```python
from build123d import *

# Parameters (mm, degrees)
SKETCH1_W           = 154
SKETCH1_H           = 41
BOSS_EXTRUDE1_DEPTH = 2
SKETCH2_R           = 1.5
CUT_EXTRUDE1_DEPTH  = 204
SKETCH3_R           = 1.5
BOSS_EXTRUDE2_DEPTH = 154
SKETCH4_W           = 12
SKETCH4_H           = 23.161381141
SKETCH4_W_2         = 3
SKETCH4_H_2         = 18.642875374
SKETCH4_H_3         = 14.783247827
SKETCH4_W_3         = 14
SKETCH4_H_4         = 17.598544921
SKETCH4_H_5         = 27.804183012
CUT_EXTRUDE2_DEPTH  = 204
SKETCH5_W           = 3
SKETCH5_H           = 13.316127407
CUT_EXTRUDE3_DEPTH  = 5
SKETCH6_W           = 8
SKETCH6_H           = 34.567606234
CUT_EXTRUDE4_DEPTH  = 1
SKETCH7_W           = 10.416873331
SKETCH7_H           = 25.160109374
BOSS_EXTRUDE3_DEPTH = 1
FILLET1_R           = 10
BOSS_EXTRUDE4_DEPTH = 2
FILLET2_R           = 2
FILLET3_R           = 2
FILLET4_R           = 0.2


with BuildPart() as part:
    # Sketch1 → Boss-Extrude1 (new body)
    with BuildSketch(Plane.XY):
        with Locations((46, -32.5)):
            Rectangle(SKETCH1_W, SKETCH1_H)
    extrude(amount=BOSS_EXTRUDE1_DEPTH)

    # Sketch2 → Cut-Extrude1 (cut)
    with BuildSketch(Plane.ZY.offset(31)):
        with Locations((-1, -17)):
            Circle(SKETCH2_R)
    extrude(amount=-CUT_EXTRUDE1_DEPTH, mode=Mode.SUBTRACT)

    # Sketch3 → Boss-Extrude2 (add)
    with BuildSketch(Plane.ZY.offset(31)):
        with BuildLine():
            Line((-2.639541446, -19.403784927), (0, -21.185182296))
            Line((0, -21.185182296), (0, -19.715731065))
            ThreePointArc((0, -19.715731065), (1.882746452, -17), (0, -14.284268935))
            Line((0, -14.284268935), (0, -13.471330145))
            Line((0, -13.471330145), (-2.092481561, -14.306696319))
            ThreePointArc((-2.092481561, -14.306696319), (-3.900693524, -16.690526404), (-2.639541446, -19.403784927))
        make_face()
        with Locations((-1.017253548, -17)):
            Circle(SKETCH3_R, mode=Mode.SUBTRACT)
    extrude(amount=-BOSS_EXTRUDE2_DEPTH)

    # Sketch4 → Cut-Extrude2 (cut)
    with BuildSketch(Plane(origin=(0, 0, 0), x_dir=(-1, 0, 0), z_dir=(0, 0, -1))):
        with Locations((22, -9.604491726)):
            Rectangle(SKETCH4_W, SKETCH4_H)
        with Locations((-80.5, -11.863744609)):
            Rectangle(SKETCH4_W_2, SKETCH4_H_2)
        with Locations((-114, -13.793558383)):
            Rectangle(SKETCH4_W, SKETCH4_H_3)
        with Locations((-103.5, -11.863744609)):
            Rectangle(SKETCH4_W_2, SKETCH4_H_2)
        with Locations((-92, -12.385909835)):
            Rectangle(SKETCH4_W_3, SKETCH4_H_4)
        with Locations((-69, -12.385909835)):
            Rectangle(SKETCH4_W_3, SKETCH4_H_4)
        with Locations((-57.5, -11.863744609)):
            Rectangle(SKETCH4_W_2, SKETCH4_H_2)
        with Locations((-46, -12.385909835)):
            Rectangle(SKETCH4_W_3, SKETCH4_H_4)
        with Locations((-34.5, -11.863744609)):
            Rectangle(SKETCH4_W_2, SKETCH4_H_2)
        with Locations((-23, -12.385909835)):
            Rectangle(SKETCH4_W_3, SKETCH4_H_4)
        with Locations((-11.5, -11.863744609)):
            Rectangle(SKETCH4_W_2, SKETCH4_H_2)
        with Locations((0, -12.385909835)):
            Rectangle(SKETCH4_W_3, SKETCH4_H_4)
        with Locations((11.5, -7.28309079)):
            Rectangle(SKETCH4_W_2, SKETCH4_H_5)
    extrude(amount=CUT_EXTRUDE2_DEPTH, mode=Mode.SUBTRACT)

    # Sketch5 → Cut-Extrude3 (cut)
    with BuildSketch(Plane(origin=(0, 0, 0), x_dir=(-1, 0, 0), z_dir=(0, 0, -1))):
        with Locations((-80.5, -11.44429523)):
            Rectangle(SKETCH5_W, SKETCH5_H)
        with Locations((-103.5, -11.44429523)):
            Rectangle(SKETCH5_W, SKETCH5_H)
        with Locations((-57.5, -11.44429523)):
            Rectangle(SKETCH5_W, SKETCH5_H)
        with Locations((-34.5, -11.44429523)):
            Rectangle(SKETCH5_W, SKETCH5_H)
        with Locations((-11.5, -11.44429523)):
            Rectangle(SKETCH5_W, SKETCH5_H)
        with Locations((11.5, -11.44429523)):
            Rectangle(SKETCH5_W, SKETCH5_H)
    extrude(amount=-CUT_EXTRUDE3_DEPTH, mode=Mode.SUBTRACT)

    # Sketch6 → Cut-Extrude4 (cut)
    with BuildSketch(Plane(origin=(0, 0, 0), x_dir=(-1, 0, 0), z_dir=(0, 0, -1))):
        with Locations((-46, -29.283803117)):
            Rectangle(SKETCH6_W, SKETCH6_H)
    extrude(amount=-CUT_EXTRUDE4_DEPTH, mode=Mode.SUBTRACT)

    # Sketch7 → Boss-Extrude3 (add)
    with BuildSketch(Plane(origin=(0, 0, 0), x_dir=(-1, 0, 0), z_dir=(0, 0, -1))):
        with Locations((-46.159585617, -34.952904223)):
            Rectangle(SKETCH7_W, SKETCH7_H)
    extrude(amount=BOSS_EXTRUDE3_DEPTH)

    # Fillet1
    # the kernel refuses this fillet: 10 mm, written as the material it takes off along each edge
    with BuildSketch(Plane(origin=(40.951148952, -11.475602177, -1), x_dir=(0, 0, 1), z_dir=(0, -1, 0)), Plane(origin=(51.368022283, -58.430206269, -1), x_dir=(0, 0, 1), z_dir=(0, 1, 0))) as fillet1_piece_1:
        with BuildLine():
            CenterArc((10, -4.358898944), FILLET1_R, 154.158067237, 25.841932763)
            Line((0, -4.358898944), (-0.2, -4.358898944))
            Line((-0.2, -4.358898944), (-0.2, 0))
            Line((-0.2, 0), (0, 0.2))
            ThreePointArc((0, 0.2), (0.5, 0.2), (0.82, 0.087177979))
            Line((0.82, 0.087177979), (1, 0))
        make_face()
    extrude(amount=46.954604092, mode=Mode.SUBTRACT)
    with BuildSketch(Plane(origin=(30.053901593, -47.53295891, -1), x_dir=(0, 0, 1), z_dir=(1, 0, 0))) as fillet1_piece_2:
        with BuildLine():
            CenterArc((10, -4.358898944), FILLET1_R, 154.158067237, 25.841932763)
            Line((0, -4.358898944), (-0.2, -4.358898944))
            Line((-0.2, -4.358898944), (-0.2, 0))
            Line((-0.2, 0), (0, 0.2))
            ThreePointArc((0, 0.2), (0.5, 0.2), (0.82, 0.087177979))
            Line((0.82, 0.087177979), (1, 0))
        make_face()
    extrude(amount=32.211368048, mode=Mode.SUBTRACT)

    # Sketch8 → Boss-Extrude4 (add)
    with BuildSketch(Plane.XY.offset(2)):
        with BuildLine():
            Line((42.287250182, -53), (49.726428085, -53))
            Line((49.726428085, -53), (49.726428085, -55.335034312))
            ThreePointArc((49.726428085, -55.335034312), (46.006839134, -57.703773476), (42.287250182, -55.335034312))
            Line((42.287250182, -55.335034312), (42.287250182, -53))
        make_face()
    extrude(amount=-BOSS_EXTRUDE4_DEPTH)

    # Fillet2
    fillet2_edges = [part.edges().sort_by_distance(p)[0] for p in [
        (49.726428085, -53, 1),
        (42.287250182, -53, 1),
    ]]
    fillet(fillet2_edges, radius=FILLET2_R)

    # Fillet3
    fillet3_edges = [part.edges().sort_by_distance(p)[0] for p in [
        (42.287250182, -55.335034312, 1),
        (49.726428085, -55.335034312, 1),
    ]]
    fillet(fillet3_edges, radius=FILLET3_R)

    # Fillet4
    fillet4_edges = [part.edges().sort_by_distance(p)[0] for p in [
        (123, -32.5, 2),
        (87.363214043, -53, 2),
        (-31, -32.5, 2),
        (-22, -12, 2),
        (0, -12, 2),
        (23, -12, 2),
        (46, -12, 2),
        (69, -12, 2),
        (92, -12, 2),
        (114, -12, 2),
        (-13, -15.051179467, 2),
        (-11.5, -18.102358934, 2),
        (-10, -15.051179467, 2),
        (10, -15.051179467, 2),
        (11.5, -18.102358934, 2),
        (13, -15.051179467, 2),
        (33, -15.051179467, 2),
        (34.5, -18.102358934, 2),
        (36, -15.051179467, 2),
        (56, -15.051179467, 2),
        (57.5, -18.102358934, 2),
        (59, -15.051179467, 2),
        (79, -15.051179467, 2),
        (80.5, -18.102358934, 2),
        (82, -15.051179467, 2),
        (103.5, -18.102358934, 2),
        (102, -15.051179467, 2),
        (105, -15.051179467, 2),
        (4.643625091, -53, 2),
        (41.666744603, -53.551899471, 2),
        (46.006839134, -57.703773476, 2),
        (50.346933665, -53.551899471, 2),
        (49.623464755, -55.453379515, 2),
        (42.390213513, -55.453379515, 2),
    ]]
    fillet(fillet4_edges, radius=FILLET4_R)


solid = part.part
```
Geometry: final body of the model. Coordinates: model frame, mm. A direction names the side the tool comes from. Coordinates: 2 decimals unless noted, no trailing zeros. Order: outer loops, then holes, each group sorted by start corner. A loop starts at its lowest first (then second) coordinate and runs counter-clockwise, first axis right, second up. Notation, with made-up numbers: M 33,21 L 40,21 A24 ccw 40,42 Z; hole C -21,38.5 d4. An arc over 180 degrees is marked long. Answer as CSV lines item,"result".
Q1. Draft query along Z for faces 1 (the cylindrical face through (54.29, -17.57, 0.37)), 2 (the cylindrical face through (91.86, -16.549, 0.413)), 3 (the cylindrical face through (-29.521, -16.647, -3.896)), 4 (the flat face through (62, -17, -3)). Return one class per face: pulls with the +Z half, pulls with the -Z half, needs draft (parallel to the pull), parting line crosses it, or undercut.
Answers:
face 1,"undercut"
face 2,"undercut"
face 3,"pulls with the -Z half"
face 4,"needs draft"
Q2. Line query: probe 1 along X at (y, z) = (-19.5, 0.7); probe 2 along Z at (x, y) = (54.75, -17); probe 3 along Y at (x, z) = (61.5, 1.35). Output: solid intervals per line, ascending. Write a range as [from, to].
Answers:
probe 1,"x = [-31, 42], [50, 123]"
probe 2,"z = [-3.92, -2.52], [0.48, 2]"
probe 3,"y = [-53, -12]"
Q3. Set-up query: faces 5 (the flat face through (30, -17, -3)), 6 (the cylindrical face through (83.479, -16.647, -3.896)), 7 (the flat face through (82, -15.6, 0.3)). Return all of +Z, -Z, +X, -X, +Y, -Y with unobstructed straight access to the full face (end or side cutting, diameter ignored); none if empty.
Answers:
face 5,"-Z, +Y, -Y"
face 6,"-Z, +X, -X"
face 7,"-Z, +Y"
Q4. Section A-A on y = -40.5. Return the cut outline in (x, z).
Answers:
outline,"M -31,0 L 40.95,0 A10 ccw 45.31,-1 L 47.01,-1 A10 ccw 51.37,0 L 123,0 L 123,1.8 A0.2 ccw 122.8,2 L -30.8,2 A0.2 ccw -31,1.8 Z; hole M 42,0 L 50,0 L 50,1 L 42,1 Z"
Q5. Section B-B on x = 80.5. Return the cut outline in (y, z).
Answers:
outline,"M -53,0 L -18.1,0 L -18.1,1.8 A0.2 ccw -18.3,2 L -52.8,2 A0.2 ccw -53,1.8 Z"
Q6. First-contact query: P1, Ø0.9, axis at x = 57.5, z = 1, coming from the +Y side; P2, Ø1, axis at x = 41, z = 1, coming from the -Y side; P3, Ø2, axis at y = -46, z = -0.5, coming from the -X side; P4, Ø8, axis at x = -7.5, y = -29.5, coming from the -Z side. Flat tips, straight axial feed; report the tip coordinate or a pass-through.
Answers:
P1,"stops at y = -18.1"
P2,"stops at y = -53.41"
P3,"stops at x = -31"
P4,"stops at z = 0"
